from build123d import *

# Parameters (mm, degrees)
F2_R     = 7.5
F2_R_2   = 5.5
F3_DEPTH = 3
F4_DEPTH = 5


# Not quite as in the source:
# - a feature names something its author has since deleted; it is built from what else it names


with BuildPart() as f3:
    # F2 (on Top) → F3 (new body)
    with BuildSketch(Plane.XY):
        with BuildLine():
            Line((40, 9.5), (0, 9.5))
            ThreePointArc((0, 9.5), (-6.7175144213, 6.7175144213), (-9.5, 0))
            ThreePointArc((-9.5, 0), (-6.7175144213, -6.7175144213), (0, -9.5))
            Line((0, -9.5), (40, -9.5))
            ThreePointArc((40, -9.5), (46.7175144213, -6.7175144213), (49.5, 0))
            ThreePointArc((49.5, 0), (46.7175144213, 6.7175144213), (40, 9.5))
        make_face()
        Circle(F2_R, mode=Mode.SUBTRACT)
        with Locations((20, 0)):
            Circle(F2_R, mode=Mode.SUBTRACT)
        with Locations((40, 0)):
            Circle(F2_R, mode=Mode.SUBTRACT)
        Circle(F2_R)
        Circle(F2_R_2, mode=Mode.SUBTRACT)
        with Locations((20, 0)):
            Circle(F2_R)
        with Locations((20, 0)):
            Circle(F2_R_2, mode=Mode.SUBTRACT)
        with Locations((40, 0)):
            Circle(F2_R)
        with Locations((40, 0)):
            Circle(F2_R_2, mode=Mode.SUBTRACT)
    extrude(amount=F3_DEPTH)

    # F2 (on Top) → F4 (join)
    with BuildSketch(Plane.XY):
        Circle(F2_R)
        Circle(F2_R_2, mode=Mode.SUBTRACT)
        with Locations((20, 0)):
            Circle(F2_R)
        with Locations((20, 0)):
            Circle(F2_R_2, mode=Mode.SUBTRACT)
        with Locations((40, 0)):
            Circle(F2_R)
        with Locations((40, 0)):
            Circle(F2_R_2, mode=Mode.SUBTRACT)
    extrude(amount=F4_DEPTH)


solid = f3.part
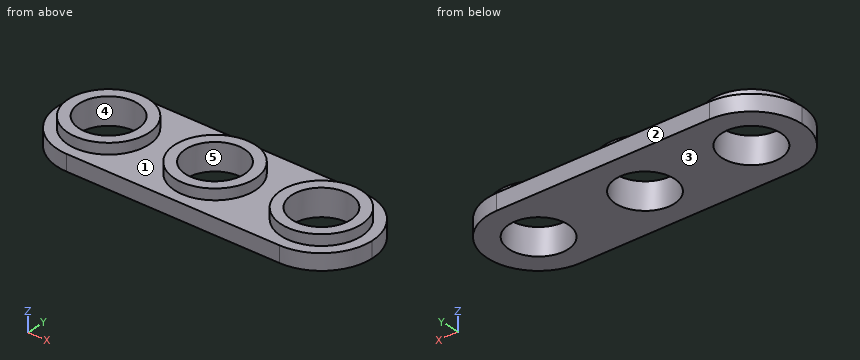
Read the model definition and answer for the solid it produces. Units are mm, in the model's axes. Face numbers are marked on the shaded views. A direction names the side the tool comes from. Round coordinates to 2 decimals unless told otherwise and drop trailing zeros. Write each loop counter-clockwise with the first axis right and the second up, starting at its lowest first coordinate (ties: lowest second). Pieces come first, ordered by that corner, then holes. Notation, with made-up numbers: (-9.5, 73) - (33.5, 73) arc R29 ccw to (33.5, 105) - close; hole circle Ø9 at (-12, -4.5). An arc over 180 degrees is marked (long way). Use a Markdown table: item, result.
(1) The part is cut by section D-D (y = 1). Write down the section's boundary in (x, z), then the cut area to 3 significant figures.
Reported:
| item | result |
|---|---|
| outline | (-9.45, 0) - (-5.41, 0) - (-5.41, 5) - (-7.43, 5) - (-7.43, 3) - (-9.45, 3) - close; (5.41, 0) - (14.59, 0) - (14.59, 5) - (12.57, 5) - (12.57, 3) - (7.43, 3) - (7.43, 5) - (5.41, 5) - close; (25.41, 0) - (34.59, 0) - (34.59, 5) - (32.57, 5) - (32.57, 3) - (27.43, 3) - (27.43, 5) - (25.41, 5) - close; (45.41, 0) - (49.45, 0) - (49.45, 3) - (47.43, 3) - (47.43, 5) - (45.41, 5) - close |
| area | 104 mm2 |
(2) The mould has two halves that part along X. Classify the marked faces 3, 4 and 5: released by +X, released by -X, zero draft, split by the parting line, or undercut.
Reported:
| item | result |
|---|---|
| face 3 | zero draft |
| face 4 | undercut |
| face 5 | undercut |
(3) Which of the six approach directions +Z, -Z, +X, -X, +Y, -Y give full straight-line access (tool end or side, diameter ignored) to the marked faces 1 and 2?
Reported:
| item | result |
|---|---|
| face 1 | +Z |
| face 2 | +Z, -Z, +X, -X, +Y |
(4) The part is cut by section C-C (z = 2.25). Write down the section's boundary in (x, y), then the cut area to 3 significant figures.
Reported:
| item | result |
|---|---|
| outline | (0, -9.5) - (40, -9.5) arc R9.5 ccw to (40, 9.5) - (0, 9.5) arc R9.5 ccw to start; hole circle Ø11 at (0, 0); hole circle Ø11 at (20, 0); hole circle Ø11 at (40, 0) |
| area | 758 mm2 |
(5) The part is cut by section A-A (z = 4.5). Write down the section's boundary in (x, y).
Reported:
| item | result |
|---|---|
| outline | circle Ø15 at (0, 0); circle Ø15 at (20, 0); circle Ø15 at (40, 0); hole circle Ø11 at (0, 0); hole circle Ø11 at (20, 0); hole circle Ø11 at (40, 0) |
(6) Straight lines are drawn through the part: line 1 along X through (y, z) = (2.25, 4.2); line 2 along Y through (x, z) = (20, 2.9); line 3 along X through (y, z) = (-3.25, 0.3). For each, find the intervals that lie inside material, in ascending order. Write a range as [from, to].
Reported:
| item | result |
|---|---|
| line 1 | [-7.15, -5.02], [5.02, 7.15], [12.85, 14.98], [25.02, 27.15], [32.85, 34.98], [45.02, 47.15] |
| line 2 | [-9.5, -5.5], [5.5, 9.5] |
| line 3 | [-8.93, -4.44], [4.44, 15.56], [24.44, 35.56], [44.44, 48.93] |
(7) Each of these flat-tipped pins is pushed along its axis until it touches: pin 1 Ø5.5 at (x, y) = (28.5, 0) entering from +Z; pin 2 Ø3 at (y, z) = (3.5, 4) entering from -X. Where does it stop, or does it pass through?
Reported:
| item | result |
|---|---|
| pin 1 | z = 5 |
| pin 2 | x = -9.2 |
(8) The part is cut by section B-B (x = 20). Write down the section's boundary in (y, z), then the cut area to 3 significant figures.
Reported:
| item | result |
|---|---|
| outline | (-9.5, 0) - (-5.5, 0) - (-5.5, 5) - (-7.5, 5) - (-7.5, 3) - (-9.5, 3) - close; (5.5, 0) - (9.5, 0) - (9.5, 3) - (7.5, 3) - (7.5, 5) - (5.5, 5) - close |
| area | 32.0 mm2 |
